Geometry: final body of the model. Coordinates: model frame, mm. Face numbers are marked on the shaded views. A direction names the side the tool comes from. Give positions to 0.01 mm unless a question says otherwise; leave off trailing zeros. Loops run counter-clockwise (first coordinate to the right, second up) from the corner with the lowest first, then second, coordinate; pieces in that order, holes last. Notation, with made-up numbers: (17.25, 47) -> (57.25, 47) arc R11 ccw to (57.25, 60) -> close; hole circle Ø11 at (42.5, -19). An arc over 180 degrees is marked (long way). One line per question, with ' | ' between items. Start each with the question number.
Item 1: Pin query (flat end, axial travel): P1, Ø6, axis at y = 1, z = 31.5, coming from the -X side; P2, Ø6, axis at x = 2, y = 2, coming from the -Z side; P3, Ø1.6, axis at x = -27.5, y = 2.5, coming from the -Z side. Return the tip coordinate at first contact, or that it passes through.
Item 2: Section C-C on x = 18. Return loops of the section in (y, z), then the cut area to 3 significant figures.
Item 3: Section A-A on z = 8. Return loops of the section in (x, y), then the cut area to 3 significant figures.
Item 4: Section D-D on y = -3.25. Return loops of the section in (x, z), then the cut area to 3 significant figures.
Item 5: Material intervals for line 1 along Z through (x, y) = (-7, 2.75); line 2 along Z through (x, y) = (-6, 11); line 3 along X through (y, z) = (-9, 23), sorted ascending. Write a range as [from, to].
Item 6: Set-up query: the marked faces 1, 2 and 3. Return all of +Z, -Z, +X, -X, +Y, -Y with unobstructed straight access to the full face (end or side cutting, diameter ignored); none if empty.
Item 7: Section B-B on y = 8.25. Return loops of the section in (x, z).
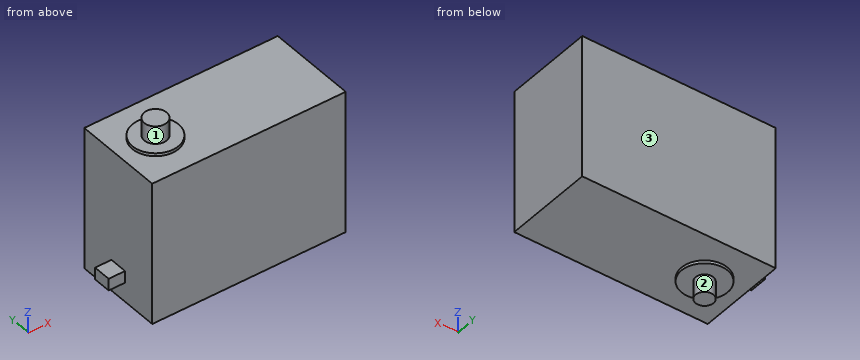
from build123d import *

# Parameters (mm, degrees)
SKETCH2_W           = 65
SKETCH2_H           = 30
BOSS_EXTRUDE1_DEPTH = 48
SKETCH3_R           = 3.75
BOSS_EXTRUDE2_DEPTH = 7
SKETCH4_R           = 7.75
BOSS_EXTRUDE3_DEPTH = 1
SKETCH5_R           = 3
BOSS_EXTRUDE6_DEPTH = 7
SKETCH7_R           = 7.75
BOSS_EXTRUDE7_DEPTH = 1
SKETCH8_W           = 4
SKETCH8_H           = 6
BOSS_EXTRUDE8_DEPTH = 5.5


with BuildPart() as part:
    # Sketch2 → Boss-Extrude1 (new body)
    with BuildSketch(Plane.XY):
        with Locations((8.357142857, 1.357142857)):
            Rectangle(SKETCH2_W, SKETCH2_H)
    extrude(amount=BOSS_EXTRUDE1_DEPTH)

    # Sketch3 → Boss-Extrude2 (add)
    with BuildSketch(Plane.XY.offset(48)):
        with Locations((-11.642857143, 1.357142857)):
            Circle(SKETCH3_R)
    extrude(amount=BOSS_EXTRUDE2_DEPTH)

    # Sketch4 → Boss-Extrude3 (add)
    with BuildSketch(Plane.XY.offset(48)):
        with Locations((-11.642857143, 1.357142857)):
            Circle(SKETCH4_R)
    extrude(amount=BOSS_EXTRUDE3_DEPTH)

    # Sketch5 → Boss-Extrude6 (add)
    with BuildSketch(Plane(origin=(0, 0, 0), x_dir=(-1, 0, 0), z_dir=(0, 0, -1))):
        with Locations((11.642857143, 1.357142857)):
            Circle(SKETCH5_R)
    extrude(amount=BOSS_EXTRUDE6_DEPTH)

    # Sketch7 → Boss-Extrude7 (add)
    with BuildSketch(Plane(origin=(0, 0, 0), x_dir=(-1, 0, 0), z_dir=(0, 0, -1))):
        with Locations((11.642857143, 1.357142857)):
            Circle(SKETCH7_R)
    extrude(amount=BOSS_EXTRUDE7_DEPTH)

    # Sketch8 → Boss-Extrude8 (add)
    with BuildSketch(Plane.ZY.offset(24.142857143)):
        with Locations((8.5, 1.357142857)):
            Rectangle(SKETCH8_W, SKETCH8_H)
    extrude(amount=BOSS_EXTRUDE8_DEPTH)


solid = part.part
Result sheet:
1) P1: stops at x = -24.14 | P2: stops at z = 0 | P3: stops at z = 6.5
2) outline: (-13.64, 0) -> (16.36, 0) -> (16.36, 48) -> (-13.64, 48) -> close | area: 1,440 mm²
3) outline: (-29.64, -1.64) -> (-24.14, -1.64) -> (-24.14, -13.64) -> (40.86, -13.64) -> (40.86, 16.36) -> (-24.14, 16.36) -> (-24.14, 4.36) -> (-29.64, 4.36) -> close | area: 1,980 mm²
4) outline: (-24.14, 0) -> (-17.87, 0) -> (-17.87, -1) -> (-5.41, -1) -> (-5.41, 0) -> (40.86, 0) -> (40.86, 48) -> (-5.41, 48) -> (-5.41, 49) -> (-17.87, 49) -> (-17.87, 48) -> (-24.14, 48) -> close | area: 3,140 mm²
5) line 1: z = [-1, 49] | line 2: z = [0, 48] | line 3: x = [-24.14, 40.86]
6) face 1: +Z | face 2: -Z | face 3: +Z, -Z, +X, -X, +Y
7) outline: (-24.14, 0) -> (-15.19, 0) -> (-15.19, -1) -> (-8.1, -1) -> (-8.1, 0) -> (40.86, 0) -> (40.86, 48) -> (-8.1, 48) -> (-8.1, 49) -> (-15.19, 49) -> (-15.19, 48) -> (-24.14, 48) -> close
